Autodesk Inventor part; units mm, degrees
ref_plane "YZ Plane" through (0, 0, 0) normal (1, 0, 0) x (0, 1, 0)
ref_plane "XZ Plane" through (0, 0, 0) normal (0, 1, 0) x (-1, 0, 0)
ref_plane "XY Plane" through (0, 0, 0) normal (0, 0, 1) x (1, 0, 0)
sketch "Sketch1" plane through (0, 0, 0) normal (0, 0, 1) x (1, 0, 0)
  circle A0 centre (0, 0) radius 25
  dimension "d0" = 50
extrude "Extrusion1" add sketch "Sketch1" along normal blind 2
sketch "Sketch2" plane through (0, 0, 2) normal (0, 0, 1) x (1, 0, 0)
  line L0 (0, 0) -> (21.2176, 12.25)
  line L1 (0, 0) -> (24.5, 0) construction
  line L2 (21.2176, 12.25) -> (23.6504, 1.0103)
  circle A0 centre (0, 0) radius 25
  line L3 (23.6504, 1.0103) -> (0, 0)
  dimension "d3" = 24.5
  dimension "d4" = 30
  dimension "d5" = 11.5
extrude "Extrusion2" cut sketch "Sketch2" against normal blind 2 contours L0 L2 L3
sketch "Sketch3" plane through (0, 0, 2) normal (0, 0, 1) x (1, 0, 0)
  point P0 (0, 0)
sketch "Sketch4" plane through (0, 0, 2) normal (0, 0, 1) x (1, 0, 0)
  line L0 (0, 0) -> (23.6504, 1.0103)
  line L1 (0, 0) -> (18.7681, 15.7483)
  line L2 (0, 0) -> (24.5, 0) construction
  line L3 (18.7681, 15.7483) -> (9.384, 22.3958)
  line L4 (9.384, 22.3958) -> (0, 0)
  dimension "d8" = 24.5
  dimension "d9" = 40
  dimension "d10" = 11.5
extrude "Extrusion3" cut sketch "Sketch4" against normal blind 2
sketch "Sketch5" plane through (0, 0, 2) normal (0, 0, 1) x (1, 0, 0)
  line L0 (23.6504, 1.0103) -> (0, 0)
  line L1 (0, 0) -> (3.6213, 24.2309)
  line L2 (0, 0) -> (24.5, 0) construction
  line L3 (3.6213, 24.2309) -> (-7.7313, 22.3958)
  line L4 (9.384, 22.3958) -> (0, 0)
  line L5 (-7.7313, 22.3958) -> (0, 0)
  dimension "d13" = 24.5
  dimension "d14" = 81.5
  dimension "d15" = 11.5
extrude "Extrusion4" cut sketch "Sketch5" against normal blind 2
sketch "Sketch6" plane through (0, 0, 2) normal (0, 0, 1) x (1, 0, 0)
  line L0 (0, 0) -> (-13.7002, 20.3114)
  line L1 (0, 0) -> (24.5, 0) construction
  line L2 (-13.7002, 20.3114) -> (-20.9994, 11.4248)
  circle A0 centre (0, 0) radius 25
  line L3 (-20.9994, 11.4248) -> (0, 0)
  dimension "d18" = 24.5
  dimension "d19" = 124
  dimension "d20" = 11.5
extrude "Extrusion5" cut sketch "Sketch6" against normal blind 2 contours L3 L2 L0
sketch "Sketch7" plane through (0, 0, 2) normal (0, 0, 1) x (1, 0, 0)
  line L0 (23.6504, 1.0103) -> (0, 0)
  line L1 (0, 0) -> (-23.6652, 6.3411)
  line L2 (0, 0) -> (24.5, 0) construction
  line L3 (-23.6652, 6.3411) -> (-22.9423, -5.1362)
  circle A0 centre (0, 0) radius 25
  line L4 (-22.9423, -5.1362) -> (0, 0)
  dimension "d23" = 24.5
  dimension "d24" = 165
  dimension "d25" = 11.5
extrude "Extrusion6" cut sketch "Sketch7" against normal blind 2 contours L4 L3 L1
sketch "Sketch8" plane through (0, 0, 2) normal (0, 0, 1) x (1, 0, 0)
  line L0 (0, 0) -> (-21.6423, -10.0067)
  line L1 (-21.6423, -10.0067) -> (-14.2585, -18.8231)
  line L2 (-14.2585, -18.8231) -> (0, 0)
  dimension "d28" = 11.5
extrude "Extrusion7" cut sketch "Sketch8" against normal blind 2
sketch "Sketch9" plane through (0, 0, 2) normal (0, 0, 1) x (1, 0, 0)
  line L0 (0, 0) -> (-21.6423, -10.0067)
  line L1 (0, 0) -> (-9.6274, -22.5292)
  line L2 (-9.6274, -22.5292) -> (1.7119, -24.4448)
  line L3 (1.7119, -24.4448) -> (0, 0)
  dimension "d31" = 24.5
  dimension "d32" = 11.5
extrude "Extrusion8" cut sketch "Sketch9" against normal blind 2
sketch "Sketch10" plane through (0, 0, 2) normal (0, 0, 1) x (1, 0, 0)
  line L0 (0, 0) -> (6.7487, -23.5)
  line L1 (6.7487, -23.5) -> (15.6191, -16.995)
  line L2 (15.6191, -16.995) -> (0, 0)
  dimension "d35" = 11
  dimension "d36" = 23.5
extrude "Extrusion9" cut sketch "Sketch10" against normal blind 2
sketch "Sketch11" plane through (0, 0, 2) normal (0, 0, 1) x (1, 0, 0)
  line L0 (0, 0) -> (-22.9423, -5.1362)
  line L1 (0, 0) -> (18.8673, -14.0098)
  line L2 (18.8673, -14.0098) -> (22.6101, -3.1358)
  line L3 (0, 0) -> (23.6504, 1.0103)
  line L4 (22.6101, -3.1358) -> (0, 0)
  dimension "d39" = 23.5
  dimension "d40" = 11.5
extrude "Extrusion10" cut sketch "Sketch11" against normal blind 2
sketch "Sketch12" plane through (0, 0, 2) normal (0, 0, 1) x (1, 0, 0)
  line L0 (-21.6423, -10.0067) -> (0, 0)
  circle A0 centre (0, 0) radius 1.5
  dimension "d43" = 3
extrude "Extrusion11" cut sketch "Sketch12" against normal blind 2
sketch "Sketch13" plane through (0, 0, 2) normal (0, 0, 1) x (1, 0, 0)
  circle A0 centre (-10.4058, 20.5939) radius 1
  point P0 (0, 0)
  dimension "d46" = 2
extrude "Extrusion12" cut sketch "Sketch13" against normal blind 2
sketch "Sketch14" plane through (0, 0, 2) normal (0, 0, 1) x (1, 0, 0)
  circle A0 centre (5.9648, 21.3776) radius 1
  point P0 (0, 0)
  dimension "d49" = 2
extrude "Extrusion13" cut sketch "Sketch14" against normal blind 2
sketch "Sketch15" plane through (0, 0, 2) normal (0, 0, 1) x (1, 0, 0)
  circle A0 centre (18.7681, 13.4535) radius 1
  point P0 (0, 0)
  dimension "d52" = 2
extrude "Extrusion14" cut sketch "Sketch15" against normal blind 2
sketch "Sketch16" plane through (0, 0, 2) normal (0, 0, 1) x (1, 0, 0)
  circle A0 centre (22.5096, -0.6531) radius 1
  point P0 (0, 0)
  dimension "d55" = 2
extrude "Extrusion15" cut sketch "Sketch16" against normal blind 2
sketch "Sketch17" plane through (0, 0, 2) normal (0, 0, 1) x (1, 0, 0)
  circle A0 centre (16.0659, -14.5855) radius 1
  point P0 (0, 0)
  dimension "d58" = 2
extrude "Extrusion16" cut sketch "Sketch17" against normal blind 2
sketch "Sketch18" plane through (0, 0, 2) normal (0, 0, 1) x (1, 0, 0)
  circle A0 centre (3.5814, -21.6389) radius 1
  point P0 (0, 0)
  dimension "d61" = 2
extrude "Extrusion17" cut sketch "Sketch18" against normal blind 2
sketch "Sketch19" plane through (0, 0, 2) normal (0, 0, 1) x (1, 0, 0)
  circle A0 centre (-11.2766, -18.5911) radius 1
  point P0 (0, 0)
  dimension "d64" = 2
extrude "Extrusion18" cut sketch "Sketch19" against normal blind 2
sketch "Sketch20" plane through (0, 0, 2) normal (0, 0, 1) x (1, 0, 0)
  circle A0 centre (-21.6423, -6.7485) radius 1
  point P0 (0, 0)
  dimension "d67" = 2
extrude "Extrusion19" cut sketch "Sketch20" against normal blind 2
sketch "Sketch21" plane through (0, 0, 2) normal (0, 0, 1) x (1, 0, 0)
  circle A0 centre (-20.5068, 8.403) radius 1
  point P0 (0, 0)
  dimension "d70" = 2
extrude "Extrusion20" cut sketch "Sketch21" against normal blind 2
sketch "Sketch22" plane through (0, 0, 2) normal (0, 0, 1) x (1, 0, 0)
  circle A0 centre (0, 0) radius 4.0832
extrude "Extrusion21" add sketch "Sketch22" along normal blind 5
properties part number "F 3"
For this review, take the finished solid that the model builds, in its own axes (mm). Coordinates: 2 decimals unless noted, no trailing zeros. Order: outer loops, then holes, each group sorted by start corner. A loop starts at its lowest first (then second) coordinate and runs counter-clockwise, first axis right, second up. Notation, with made-up numbers: (88, -20.75) - (109, -20.75) arc R21 cw to (109, 14.25) - close; hole circle Ø2 at (35, 47). An arc over 180 degrees is marked (long way). Answer as CSV lines item,"result". Start each with the question number.
1) To check wall thickness, follow line 1 along Y through (x, z) = (14, 1.75); line 2 along Y through (x, z) = (16, 0.75); line 3 along X through (y, z) = (14, 1.25). State the ranges of each line that lie inside material, in increasing order. Write a range as [from, to].
2) Add section C-C (z = 3.25). State the section outline as (x, y) points, then the cut area to 3 significant figures.
3) Draft analysis for pull direction Y (two halves, no side actions). For faces 1 (the cylindrical face through (23.846, -7.509, 0.986)), 2 (the flat face through (-4.16, 12.05, 1.01)), 3 (the flat face through (-4, 2, 2)), 4 (the flat face through (-5.045, -11.806, 1.014)), state which applies: +Y half, -Y half, draft (parallel to the pull), parting line (faces both ways), or undercut.
4) Add section A-A (x = 6). State the section outline as (y, z) points, then the cut area to 3 significant figures.
5) Add section B-B (y = 19). State the section outline as (x, z) points.
6) Insertion check: P1, Ø3, axis at x = 22.51, y = -0.65, coming from the +Z side; P2, Ø1.5, axis at y = 2, z = 3, coming from the +X side; P3, Ø1, axis at y = -1.5, z = 5, coming from the +X side. Each pin has a flat end and moves straight along its axis. Give the tip position at first contact, or say it passes through.
Result:
1,line 1,"[-20.71, -18.18], [-15.23, -10.4], [-1.94, 0.6], [8.08, 11.75], [19.13, 20.71]"
1,line 2,"[-19.21, -15.58], [-13.59, -11.88], [-2.22, 0.68], [9.24, 13.43], [17.71, 19.21]"
1,line 3,"[-20.71, -18.88], [-9.44, -4.83], [2.09, 5.87], [16.68, 17.93], [19.61, 20.71]"
2,outline,"circle Ø8.17 at (0, 0)"
2,area,"52.4 mm^2"
3,face 1,"parting line"
3,face 2,"undercut"
3,face 3,"draft"
3,face 4,"undercut"
4,outline,"(-24.27, 0) - (-20.89, 0) - (-20.89, 2) - (-24.27, 2) - close; (-6.53, 0) - (-4.46, 0) - (-4.46, 2) - (-6.53, 2) - close; (-0.83, 0) - (0.26, 0) - (0.26, 2) - (-0.83, 2) - close; (3.46, 0) - (5.03, 0) - (5.03, 2) - (3.46, 2) - close; (14.32, 0) - (20.38, 0) - (20.38, 2) - (14.32, 2) - close; (22.38, 0) - (24.27, 0) - (24.27, 2) - (22.38, 2) - close"
4,area,"32.1 mm^2"
5,outline,"(-16.25, 0) - (-14.78, 0) - (-14.78, 2) - (-16.25, 2) - close; (-12.82, 0) - (-6.56, 0) - (-6.56, 2) - (-12.82, 2) - close; (2.84, 0) - (7.96, 0) - (7.96, 2) - (2.84, 2) - close; (14.18, 0) - (16.25, 0) - (16.25, 2) - (14.18, 2) - close"
6,P1,"z = 2"
6,P2,"x = 3.89"
6,P3,"x = 3.96"
